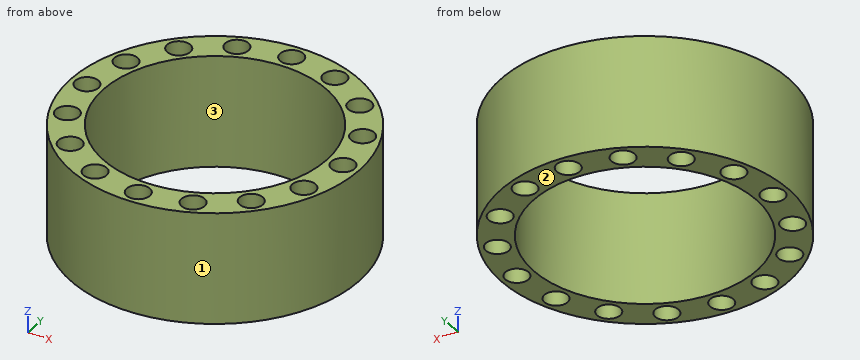
```python
from build123d import *

# Parameters (mm, degrees)
SKETCH_1_R                = 31
SKETCH_1_R_2              = 24
EXTRUDE_1_DEPTH           = 24
HOLE_WIZARD_M3_1_D        = 3.4
SKETCH_7_R                = 2.5
CUT_EXTRUDE_3_DEPTH       = 6
PATTERN_CIRCULAR_3_COUNT  = 16
MIRROR_1_COPY_1_D         = 3.4
MIRROR_1_COPY_2_D         = 3.4
MIRROR_1_COPY_3_D         = 3.4
MIRROR_1_COPY_4_D         = 3.4
MIRROR_1_COPY_5_D         = 3.4
MIRROR_1_COPY_6_D         = 3.4
MIRROR_1_COPY_7_D         = 3.4
MIRROR_1_COPY_8_D         = 3.4
MIRROR_1_COPY_9_D         = 3.4
MIRROR_1_COPY_10_D        = 3.4
MIRROR_1_COPY_11_D        = 3.4
MIRROR_1_COPY_12_D        = 3.4
MIRROR_1_COPY_13_D        = 3.4
MIRROR_1_COPY_14_D        = 3.4
MIRROR_1_COPY_15_D        = 3.4
MIRROR_1_COPY_16_SKETCH_R = 2.5
MIRROR_1_COPY_16_DEPTH    = 6
MIRROR_1_COPY_17_SKETCH_R = 2.5
MIRROR_1_COPY_17_DEPTH    = 6
MIRROR_1_COPY_18_SKETCH_R = 2.5
MIRROR_1_COPY_18_DEPTH    = 6
MIRROR_1_COPY_19_SKETCH_R = 2.5
MIRROR_1_COPY_19_DEPTH    = 6
MIRROR_1_COPY_20_SKETCH_R = 2.5
MIRROR_1_COPY_20_DEPTH    = 6
MIRROR_1_COPY_21_SKETCH_R = 2.5
MIRROR_1_COPY_21_DEPTH    = 6
MIRROR_1_COPY_22_SKETCH_R = 2.5
MIRROR_1_COPY_22_DEPTH    = 6
MIRROR_1_COPY_23_SKETCH_R = 2.5
MIRROR_1_COPY_23_DEPTH    = 6
MIRROR_1_COPY_24_SKETCH_R = 2.5
MIRROR_1_COPY_24_DEPTH    = 6
MIRROR_1_COPY_25_SKETCH_R = 2.5
MIRROR_1_COPY_25_DEPTH    = 6
MIRROR_1_COPY_26_SKETCH_R = 2.5
MIRROR_1_COPY_26_DEPTH    = 6
MIRROR_1_COPY_27_SKETCH_R = 2.5
MIRROR_1_COPY_27_DEPTH    = 6
MIRROR_1_COPY_28_SKETCH_R = 2.5
MIRROR_1_COPY_28_DEPTH    = 6
MIRROR_1_COPY_29_SKETCH_R = 2.5
MIRROR_1_COPY_29_DEPTH    = 6
MIRROR_1_COPY_30_SKETCH_R = 2.5
MIRROR_1_COPY_30_DEPTH    = 6
MIRROR_1_COPY_31_D        = 3.4


with BuildPart() as part:
    # ｽｹｯﾁ1 → ﾎﾞｽ - 押し出し1 (new body)
    with BuildSketch(Plane.XY):
        Circle(SKETCH_1_R)
        Circle(SKETCH_1_R_2, mode=Mode.SUBTRACT)
    extrude(amount=EXTRUDE_1_DEPTH)

    # M3 すきま穴1 (through all)
    with Locations(Plane.XY.offset(24)):
        with Locations((0, 27.5)):
            hole_wizard_m3_1 = Hole(HOLE_WIZARD_M3_1_D / 2)

    # ｽｹｯﾁ7 → ｶｯﾄ - 押し出し3 (cut)
    with BuildSketch(Plane.XY.offset(24)):
        with Locations((0, 27.5)):
            Circle(SKETCH_7_R)
    cut_extrude_3 = extrude(amount=-CUT_EXTRUDE_3_DEPTH, mode=Mode.SUBTRACT)

    # 円形ﾊﾟﾀｰﾝ3: M3 すきま穴1, ｶｯﾄ - 押し出し3 ×16 about axis
    pattern_circular_3_axis = Axis((0, 0, 0), (0, 0, 1))
    for i in range(1, PATTERN_CIRCULAR_3_COUNT):
        add(hole_wizard_m3_1.rotate(pattern_circular_3_axis, i * 360 / PATTERN_CIRCULAR_3_COUNT), mode=Mode.SUBTRACT)
        add(cut_extrude_3.rotate(pattern_circular_3_axis, i * 360 / PATTERN_CIRCULAR_3_COUNT), mode=Mode.SUBTRACT)

    # ﾐﾗｰ1: ｶｯﾄ - 押し出し3 across plane
    add(cut_extrude_3.mirror(Plane(origin=(0, 0, 12), x_dir=(1, 0, 0), z_dir=(0, 0, -1))), mode=Mode.SUBTRACT)

    # ﾐﾗｰ1 copy 1 (through all)
    with Locations(Plane(origin=(0, 0, 0), x_dir=(0.923879533, 0.382683432, 0), z_dir=(0, 0, -1))):
        with Locations((0, -27.5)):
            Hole(MIRROR_1_COPY_1_D / 2)

    # ﾐﾗｰ1 copy 2 (through all)
    with Locations(Plane(origin=(0, 0, 0), x_dir=(0.707106781, 0.707106781, 0), z_dir=(0, 0, -1))):
        with Locations((0, -27.5)):
            Hole(MIRROR_1_COPY_2_D / 2)

    # ﾐﾗｰ1 copy 3 (through all)
    with Locations(Plane(origin=(0, 0, 0), x_dir=(0.382683432, 0.923879533, 0), z_dir=(0, 0, -1))):
        with Locations((0, -27.5)):
            Hole(MIRROR_1_COPY_3_D / 2)

    # ﾐﾗｰ1 copy 4 (through all)
    with Locations(Plane.YX):
        with Locations((0, -27.5)):
            Hole(MIRROR_1_COPY_4_D / 2)

    # ﾐﾗｰ1 copy 5 (through all)
    with Locations(Plane(origin=(0, 0, 0), x_dir=(-0.382683432, 0.923879533, 0), z_dir=(0, 0, -1))):
        with Locations((0, -27.5)):
            Hole(MIRROR_1_COPY_5_D / 2)

    # ﾐﾗｰ1 copy 6 (through all)
    with Locations(Plane(origin=(0, 0, 0), x_dir=(-0.707106781, 0.707106781, 0), z_dir=(0, 0, -1))):
        with Locations((0, -27.5)):
            Hole(MIRROR_1_COPY_6_D / 2)

    # ﾐﾗｰ1 copy 7 (through all)
    with Locations(Plane(origin=(0, 0, 0), x_dir=(-0.923879533, 0.382683432, 0), z_dir=(0, 0, -1))):
        with Locations((0, -27.5)):
            Hole(MIRROR_1_COPY_7_D / 2)

    # ﾐﾗｰ1 copy 8 (through all)
    with Locations(Plane(origin=(0, 0, 0), x_dir=(-1, 0, 0), z_dir=(0, 0, -1))):
        with Locations((0, -27.5)):
            Hole(MIRROR_1_COPY_8_D / 2)

    # ﾐﾗｰ1 copy 9 (through all)
    with Locations(Plane(origin=(0, 0, 0), x_dir=(-0.923879533, -0.382683432, 0), z_dir=(0, 0, -1))):
        with Locations((0, -27.5)):
            Hole(MIRROR_1_COPY_9_D / 2)

    # ﾐﾗｰ1 copy 10 (through all)
    with Locations(Plane(origin=(0, 0, 0), x_dir=(-0.707106781, -0.707106781, 0), z_dir=(0, 0, -1))):
        with Locations((0, -27.5)):
            Hole(MIRROR_1_COPY_10_D / 2)

    # ﾐﾗｰ1 copy 11 (through all)
    with Locations(Plane(origin=(0, 0, 0), x_dir=(-0.382683432, -0.923879533, 0), z_dir=(0, 0, -1))):
        with Locations((0, -27.5)):
            Hole(MIRROR_1_COPY_11_D / 2)

    # ﾐﾗｰ1 copy 12 (through all)
    with Locations(Plane(origin=(0, 0, 0), x_dir=(0, -1, 0), z_dir=(0, 0, -1))):
        with Locations((0, -27.5)):
            Hole(MIRROR_1_COPY_12_D / 2)

    # ﾐﾗｰ1 copy 13 (through all)
    with Locations(Plane(origin=(0, 0, 0), x_dir=(0.382683432, -0.923879533, 0), z_dir=(0, 0, -1))):
        with Locations((0, -27.5)):
            Hole(MIRROR_1_COPY_13_D / 2)

    # ﾐﾗｰ1 copy 14 (through all)
    with Locations(Plane(origin=(0, 0, 0), x_dir=(0.707106781, -0.707106781, 0), z_dir=(0, 0, -1))):
        with Locations((0, -27.5)):
            Hole(MIRROR_1_COPY_14_D / 2)

    # ﾐﾗｰ1 copy 15 (through all)
    with Locations(Plane(origin=(0, 0, 0), x_dir=(0.923879533, -0.382683432, 0), z_dir=(0, 0, -1))):
        with Locations((0, -27.5)):
            Hole(MIRROR_1_COPY_15_D / 2)

    # ﾐﾗｰ1 copy 16 sketch → ﾐﾗｰ1 copy 16 (cut)
    with BuildSketch(Plane(origin=(0, 0, 0), x_dir=(0.923879533, 0.382683432, 0), z_dir=(0, 0, -1))):
        with Locations((0, -27.5)):
            Circle(MIRROR_1_COPY_16_SKETCH_R)
    extrude(amount=-MIRROR_1_COPY_16_DEPTH, mode=Mode.SUBTRACT)

    # ﾐﾗｰ1 copy 17 sketch → ﾐﾗｰ1 copy 17 (cut)
    with BuildSketch(Plane(origin=(0, 0, 0), x_dir=(0.707106781, 0.707106781, 0), z_dir=(0, 0, -1))):
        with Locations((0, -27.5)):
            Circle(MIRROR_1_COPY_17_SKETCH_R)
    extrude(amount=-MIRROR_1_COPY_17_DEPTH, mode=Mode.SUBTRACT)

    # ﾐﾗｰ1 copy 18 sketch → ﾐﾗｰ1 copy 18 (cut)
    with BuildSketch(Plane(origin=(0, 0, 0), x_dir=(0.382683432, 0.923879533, 0), z_dir=(0, 0, -1))):
        with Locations((0, -27.5)):
            Circle(MIRROR_1_COPY_18_SKETCH_R)
    extrude(amount=-MIRROR_1_COPY_18_DEPTH, mode=Mode.SUBTRACT)

    # ﾐﾗｰ1 copy 19 sketch → ﾐﾗｰ1 copy 19 (cut)
    with BuildSketch(Plane.YX):
        with Locations((0, -27.5)):
            Circle(MIRROR_1_COPY_19_SKETCH_R)
    extrude(amount=-MIRROR_1_COPY_19_DEPTH, mode=Mode.SUBTRACT)

    # ﾐﾗｰ1 copy 20 sketch → ﾐﾗｰ1 copy 20 (cut)
    with BuildSketch(Plane(origin=(0, 0, 0), x_dir=(-0.382683432, 0.923879533, 0), z_dir=(0, 0, -1))):
        with Locations((0, -27.5)):
            Circle(MIRROR_1_COPY_20_SKETCH_R)
    extrude(amount=-MIRROR_1_COPY_20_DEPTH, mode=Mode.SUBTRACT)

    # ﾐﾗｰ1 copy 21 sketch → ﾐﾗｰ1 copy 21 (cut)
    with BuildSketch(Plane(origin=(0, 0, 0), x_dir=(-0.707106781, 0.707106781, 0), z_dir=(0, 0, -1))):
        with Locations((0, -27.5)):
            Circle(MIRROR_1_COPY_21_SKETCH_R)
    extrude(amount=-MIRROR_1_COPY_21_DEPTH, mode=Mode.SUBTRACT)

    # ﾐﾗｰ1 copy 22 sketch → ﾐﾗｰ1 copy 22 (cut)
    with BuildSketch(Plane(origin=(0, 0, 0), x_dir=(-0.923879533, 0.382683432, 0), z_dir=(0, 0, -1))):
        with Locations((0, -27.5)):
            Circle(MIRROR_1_COPY_22_SKETCH_R)
    extrude(amount=-MIRROR_1_COPY_22_DEPTH, mode=Mode.SUBTRACT)

    # ﾐﾗｰ1 copy 23 sketch → ﾐﾗｰ1 copy 23 (cut)
    with BuildSketch(Plane(origin=(0, 0, 0), x_dir=(-1, 0, 0), z_dir=(0, 0, -1))):
        with Locations((0, -27.5)):
            Circle(MIRROR_1_COPY_23_SKETCH_R)
    extrude(amount=-MIRROR_1_COPY_23_DEPTH, mode=Mode.SUBTRACT)

    # ﾐﾗｰ1 copy 24 sketch → ﾐﾗｰ1 copy 24 (cut)
    with BuildSketch(Plane(origin=(0, 0, 0), x_dir=(-0.923879533, -0.382683432, 0), z_dir=(0, 0, -1))):
        with Locations((0, -27.5)):
            Circle(MIRROR_1_COPY_24_SKETCH_R)
    extrude(amount=-MIRROR_1_COPY_24_DEPTH, mode=Mode.SUBTRACT)

    # ﾐﾗｰ1 copy 25 sketch → ﾐﾗｰ1 copy 25 (cut)
    with BuildSketch(Plane(origin=(0, 0, 0), x_dir=(-0.707106781, -0.707106781, 0), z_dir=(0, 0, -1))):
        with Locations((0, -27.5)):
            Circle(MIRROR_1_COPY_25_SKETCH_R)
    extrude(amount=-MIRROR_1_COPY_25_DEPTH, mode=Mode.SUBTRACT)

    # ﾐﾗｰ1 copy 26 sketch → ﾐﾗｰ1 copy 26 (cut)
    with BuildSketch(Plane(origin=(0, 0, 0), x_dir=(-0.382683432, -0.923879533, 0), z_dir=(0, 0, -1))):
        with Locations((0, -27.5)):
            Circle(MIRROR_1_COPY_26_SKETCH_R)
    extrude(amount=-MIRROR_1_COPY_26_DEPTH, mode=Mode.SUBTRACT)

    # ﾐﾗｰ1 copy 27 sketch → ﾐﾗｰ1 copy 27 (cut)
    with BuildSketch(Plane(origin=(0, 0, 0), x_dir=(0, -1, 0), z_dir=(0, 0, -1))):
        with Locations((0, -27.5)):
            Circle(MIRROR_1_COPY_27_SKETCH_R)
    extrude(amount=-MIRROR_1_COPY_27_DEPTH, mode=Mode.SUBTRACT)

    # ﾐﾗｰ1 copy 28 sketch → ﾐﾗｰ1 copy 28 (cut)
    with BuildSketch(Plane(origin=(0, 0, 0), x_dir=(0.382683432, -0.923879533, 0), z_dir=(0, 0, -1))):
        with Locations((0, -27.5)):
            Circle(MIRROR_1_COPY_28_SKETCH_R)
    extrude(amount=-MIRROR_1_COPY_28_DEPTH, mode=Mode.SUBTRACT)

    # ﾐﾗｰ1 copy 29 sketch → ﾐﾗｰ1 copy 29 (cut)
    with BuildSketch(Plane(origin=(0, 0, 0), x_dir=(0.707106781, -0.707106781, 0), z_dir=(0, 0, -1))):
        with Locations((0, -27.5)):
            Circle(MIRROR_1_COPY_29_SKETCH_R)
    extrude(amount=-MIRROR_1_COPY_29_DEPTH, mode=Mode.SUBTRACT)

    # ﾐﾗｰ1 copy 30 sketch → ﾐﾗｰ1 copy 30 (cut)
    with BuildSketch(Plane(origin=(0, 0, 0), x_dir=(0.923879533, -0.382683432, 0), z_dir=(0, 0, -1))):
        with Locations((0, -27.5)):
            Circle(MIRROR_1_COPY_30_SKETCH_R)
    extrude(amount=-MIRROR_1_COPY_30_DEPTH, mode=Mode.SUBTRACT)

    # ﾐﾗｰ1 copy 31 (through all)
    with Locations(Plane(origin=(0, 0, 0), x_dir=(1, 0, 0), z_dir=(0, 0, -1))):
        with Locations((0, -27.5)):
            Hole(MIRROR_1_COPY_31_D / 2)


solid = part.part
```
Here's how the part is built. I have some questions about the finished solid (model axes, mm). Face numbers are marked on the shaded views. Give positions to 0.01 mm unless a question says otherwise; leave off trailing zeros. Write each question's results on one line, items separated by ' | '.
Item 1: Suppose I cut it at A-A on y = 0. Give the number of separate pieces and of enclosed holes in the cut face, plus the area to 3 significant figures.
Output:
separate pieces: 4 | enclosed holes: 0 | area: 134 mm^2
Item 2: We'd pull the mould along Y, two halves only. Please class the marked faces 1, 2 and 3: pulls with the +Y half, pulls with the -Y half, needs draft (parallel to the pull), parting line crosses it, or undercut.
Output:
face 1: parting line crosses it | face 2: needs draft | face 3: undercut
Item 3: For pin 1 Ø3 at (y, z) = (-20.5, 11.5) entering from +X; pin 2 Ø6 at (x, y) = (10.52, -25.41) entering from +Z; pin 3 Ø4 at (x, y) = (-19.45, -19.45) entering from -Z; pin 4 Ø4 at (x, y) = (27.5, 0) entering from +Z, each with a flat end and sliding along its axis, tell me the tip position at first contact or that it passes through.
Output:
pin 1: stops at x = 24.49 | pin 2: stops at z = 24 | pin 3: stops at z = 6 | pin 4: stops at z = 18
Item 4: If I drill on L1, parallel to Y at x = -26.5, z = 7; L2, parallel to X at y = -1.5, z = 6.5; L3, parallel to X at y = 25, z = 13, over which ranges is the centre line in solid material (lowest first)?
Output:
L1: y = -16.09 to -11.83, -9.22 to -1.37, 1.37 to 9.22, 11.83 to 16.09 | L2: x = -30.96 to -28.3, -26.7 to -23.95, 23.95 to 26.7, 28.3 to 30.96 | L3: x = -18.33 to -12.17, -8.87 to 8.87, 12.17 to 18.33
